from build123d import *

# Parameters (mm, degrees)
SKETCH1_W           = 26.4
SKETCH1_H           = 26.4
SKETCH1_W_2         = 20.4
SKETCH1_H_2         = 20.4
BOSS_EXTRUDE1_DEPTH = 40
SKETCH2_W           = 26.4
SKETCH2_H           = 26.4
BOSS_EXTRUDE2_DEPTH = 3
SKETCH3_W           = 20.4
SKETCH3_H           = 40
CUT_EXTRUDE1_DEPTH  = 3
SKETCH4_R           = 1.25
CUT_EXTRUDE2_DEPTH  = 3
SKETCH5_W           = 26.4
SKETCH5_H           = 43
CUT_EXTRUDE3_DEPTH  = 10


with BuildPart() as part:
    # Sketch1 → Boss-Extrude1 (new body)
    with BuildSketch(Plane.XY):
        Rectangle(SKETCH1_W, SKETCH1_H)
        Rectangle(SKETCH1_W_2, SKETCH1_H_2, mode=Mode.SUBTRACT)
    extrude(amount=BOSS_EXTRUDE1_DEPTH)

    # Sketch2 → Boss-Extrude2 (add)
    with BuildSketch(Plane(origin=(0, 0, 0), x_dir=(-1, 0, 0), z_dir=(0, 0, -1))):
        Rectangle(SKETCH2_W, SKETCH2_H)
    extrude(amount=BOSS_EXTRUDE2_DEPTH)

    # Sketch3 → Cut-Extrude1 (cut)
    with BuildSketch(Plane.XZ.offset(13.2)):
        with Locations((0, 20)):
            Rectangle(SKETCH3_W, SKETCH3_H)
    extrude(amount=-CUT_EXTRUDE1_DEPTH, mode=Mode.SUBTRACT)

    # Sketch4 → Cut-Extrude2 (cut)
    with BuildSketch(Plane(origin=(0, 13.2, 0), x_dir=(1, 0, 0), z_dir=(0, 1, 0))):
        with Locations(Location((0, -15, 0), (0, 0, 270))):
            Circle(SKETCH4_R)
        with Locations(Location((0, -30, 0), (0, 0, 270))):
            Circle(SKETCH4_R)
    extrude(amount=-CUT_EXTRUDE2_DEPTH, mode=Mode.SUBTRACT)

    # Sketch5 → Cut-Extrude3 (cut)
    with BuildSketch(Plane.XZ.offset(13.2)):
        with Locations((0, 18.5)):
            Rectangle(SKETCH5_W, SKETCH5_H)
    extrude(amount=-CUT_EXTRUDE3_DEPTH, mode=Mode.SUBTRACT)


solid = part.part
Source: CAD feature listing. Evaluate the final solid. Frame: model axes, mm. A direction names the side the tool comes from. Give positions to 0.01 mm unless a question says otherwise; leave off trailing zeros. Write each loop counter-clockwise with the first axis right and the second up, starting at its lowest first coordinate (ties: lowest second). Pieces come first, ordered by that corner, then holes. Notation, with made-up numbers: (33, 28.5) -> (86, 28.5) arc R28 ccw to (86, 49.5) -> close; hole circle Ø3 at (20, 37.5). An arc over 180 degrees is marked (long way). Return JSON: item names as keys, results as strings. Group by question number.
1. Section B-B, the plane z = 15. Output: boundary loops of the cut face in (x, y).
2. Access query for faces 1 (the face through (-13.2, 5, 19)), 2 (the face through (0, 10.2, 20)). Directions: +Z, -Z, +X, -X, +Y, -Y. A direction counts if a zero-diameter tool reaches every point of the face in a straight line with its end or side. Return the directions, or none.
3. Mould query, pull axis Z, two halves, no side actions, for faces 3 (the face through (0, 13.2, 19)), 4 (the face through (0, 5, -3)), 5 (the face through (0.05, 11.72, 13.75)), 6 (the face through (-0.479, 11.721, 31.155)). Classes: +Z half, -Z half, draft (parallel to the pull), parting line (faces both ways), or undercut.
4. Section D-D, the plane z = 33. Output: boundary loops of the cut face in (x, y).
5. Pin query (flat end, axial travel): pin 1 Ø1.5 at (x, z) = (4, 8) entering from -Y; pin 2 Ø2 at (x, z) = (0, 30) entering from +Y. Return the tip coordinate at first contact, or that it passes through.
6. Section C-C, the plane y = 8.25. Output: boundary loops of the cut face in (x, z), then the cut area to 3 significant figures.
7. Material intervals for line 1 (X direction, y = 12.05, z = 30); line 2 (X direction, y = 3.5, z = 32); line 3 (Z direction, x = -0.5, y = 10.5), sorted ascending. Write a range as from..to.
8. Section A-A, the plane x = 0. Output: boundary loops of the cut face in (y, z).
Determined:
{
 "1": {"outline": "(-13.2, -3.2) -> (-10.2, -3.2) -> (-10.2, 10.2) -> (-1.25, 10.2) -> (-1.25, 13.2) -> (-13.2, 13.2) -> close; (1.25, 10.2) -> (10.2, 10.2) -> (10.2, -3.2) -> (13.2, -3.2) -> (13.2, 13.2) -> (1.25, 13.2) -> close"},
 "2": {"face 1": "+Z, -Z, -X, +Y, -Y", "face 2": "+Z, -Y"},
 "3": {"face 3": "draft", "face 4": "-Z half", "face 5": "undercut", "face 6": "undercut"},
 "4": {"outline": "(-13.2, -3.2) -> (-10.2, -3.2) -> (-10.2, 10.2) -> (10.2, 10.2) -> (10.2, -3.2) -> (13.2, -3.2) -> (13.2, 13.2) -> (-13.2, 13.2) -> close"},
 "5": {"pin 1": "stops at y = 10.2", "pin 2": "passes through"},
 "6": {"outline": "(-13.2, -3) -> (13.2, -3) -> (13.2, 40) -> (10.2, 40) -> (10.2, 0) -> (-10.2, 0) -> (-10.2, 40) -> (-13.2, 40) -> close", "area": "319 mm2"},
 "7": {"line 1": "x = -13.2..-1.25, 1.25..13.2", "line 2": "x = -13.2..-10.2, 10.2..13.2", "line 3": "z = -3..13.85, 16.15..28.85, 31.15..40"},
 "8": {"outline": "(-3.2, -3) -> (13.2, -3) -> (13.2, 13.75) -> (10.2, 13.75) -> (10.2, 0) -> (-3.2, 0) -> close; (10.2, 16.25) -> (13.2, 16.25) -> (13.2, 28.75) -> (10.2, 28.75) -> close; (10.2, 31.25) -> (13.2, 31.25) -> (13.2, 40) -> (10.2, 40) -> close"}
}
